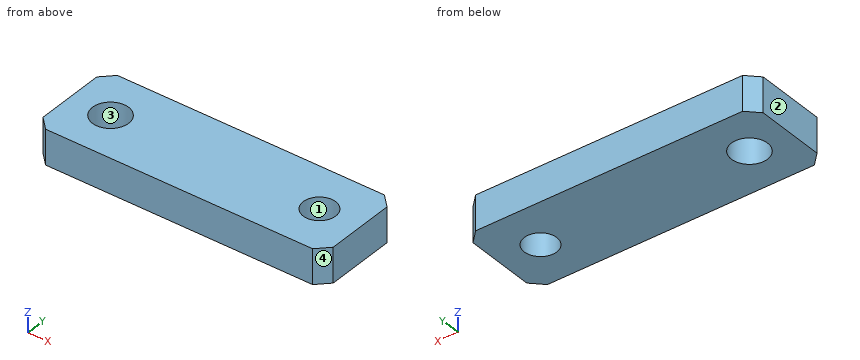
from build123d import *

# Parameters (mm, degrees)
SKETCH1_W           = 50
SKETCH1_H           = 16
SKETCH1_R           = 3.112420157
SKETCH1_R_2         = 2.795165179
BOSS_EXTRUDE1_DEPTH = 6
CHAMFER1_SIZE       = 2


with BuildPart() as part:
    # Sketch1 → Boss-Extrude1 (new body)
    with BuildSketch(Plane.XY):
        Rectangle(SKETCH1_W, SKETCH1_H)
        with Locations((-18, 0)):
            Circle(SKETCH1_R, mode=Mode.SUBTRACT)
        with Locations((18, 0)):
            Circle(SKETCH1_R_2, mode=Mode.SUBTRACT)
    extrude(amount=BOSS_EXTRUDE1_DEPTH)

    # Chamfer1
    chamfer1_edges = [part.edges().sort_by_distance(p)[0] for p in [
        (25, -8, 3),
        (-25, -8, 3),
        (-25, 8, 3),
        (25, 8, 3),
    ]]
    chamfer(chamfer1_edges, length=CHAMFER1_SIZE)


solid = part.part
For this review, take the finished solid that the model builds, in its own axes (mm). Face numbers are marked on the shaded views. Round coordinates to 2 decimals unless told otherwise and drop trailing zeros. Write each loop counter-clockwise with the first axis right and the second up, starting at its lowest first coordinate (ties: lowest second). Pieces come first, ordered by that corner, then holes. Notation, with made-up numbers: (59, 63.5) - (108, 63.5) arc R22 ccw to (108, 99.5) - close; hole circle Ø10 at (-27.5, 58). An arc over 180 degrees is marked (long way). Write item = value, one per line. Start each with the question number.
1. Consider section C-C on y = 0. State the section outline as (x, z) points.
2. For pin 1 Ø2 at (x, y) = (2.5, -4) entering from -Z; pin 2 Ø5 at (x, y) = (18, 0) entering from +Z, all flat-tipped, find the tip position at first contact; note any pin that passes through.
3. Consider section B-B on z = 2.9. State the section outline as (x, y) points, plus the area to 3 significant figures.
4. Consider section D-D on x = -18. State the section outline as (y, z) points, plus the area to 3 significant figures.
5. Draft analysis for pull direction Y (two halves, no side actions). For the marked faces 1, 2, 3 and 4, state which applies: released by +Y, released by -Y, zero draft, split by the parting line, or undercut.
6. Consider section A-A on x = 18. State the section outline as (y, z) points, plus the area to 3 significant figures.
7. Wall thickness on L1, parallel to Y at x = 18, z = 4.45; L2, parallel to X at y = -2, z = 4.5; L3, parallel to X at y = -1, z = 1.7: over which ranges is each line inside the solid? List them lowest first.
Evaluation:
q1.outline = (-25, 0) - (-21.11, 0) - (-21.11, 6) - (-25, 6) - close; (-14.89, 0) - (15.2, 0) - (15.2, 6) - (-14.89, 6) - close; (20.8, 0) - (25, 0) - (25, 6) - (20.8, 6) - close
q2.pin_1 = 0
q2.pin_2 = through
q3.outline = (-25, -6) - (-23, -8) - (23, -8) - (25, -6) - (25, 6) - (23, 8) - (-23, 8) - (-25, 6) - close; hole circle Ø6.22 at (-18, 0); hole circle Ø5.59 at (18, 0)
q3.area = 737 mm2
q4.outline = (-8, 0) - (-3.11, 0) - (-3.11, 6) - (-8, 6) - close; (3.11, 0) - (8, 0) - (8, 6) - (3.11, 6) - close
q4.area = 58.7 mm2
q5.face_1 = undercut
q5.face_2 = zero draft
q5.face_3 = undercut
q5.face_4 = released by -Y
q6.outline = (-8, 0) - (-2.8, 0) - (-2.8, 6) - (-8, 6) - close; (2.8, 0) - (8, 0) - (8, 6) - (2.8, 6) - close
q6.area = 62.5 mm2
q7.L1 = -8 to -2.8, 2.8 to 8
q7.L2 = -25 to -20.38, -15.62 to 16.05, 19.95 to 25
q7.L3 = -25 to -20.95, -15.05 to 15.39, 20.61 to 25
